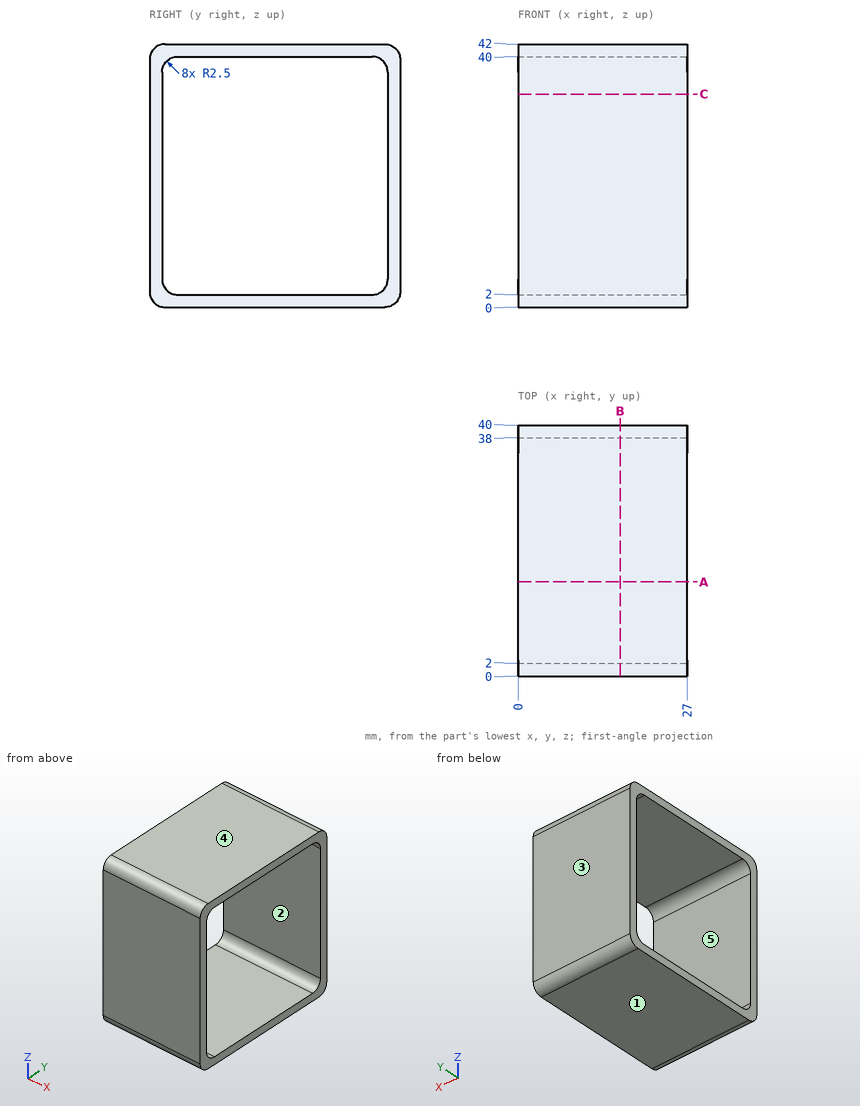
The figure shows three views and two pictorial views of one solid part (mm, origin at its lowest corner). Answer the questions. A direction names the side the tool comes from. Give positions to 0.01 mm unless a question says otherwise; leave off trailing zeros. Loops run counter-clockwise (first coordinate to the right, second up) from the corner with the lowest first, then second, coordinate; pieces in that order, holes last. Notation, with made-up numbers: (27, 35.5) -> (45, 35.5) arc R22 cw to (45, 44.5) -> close; hole circle Ø1 at (1.25, 76.5). An arc over 180 degrees is marked (long way). Put each result on its own line as item: value. Start each with the question number.
Item 1: The part is cut by section C-C (z = 34). Give the vertices of the cut face in (x, y).
Item 2: This flat-tipped pin is pushed along its axis until it touches: P1, Ø8, axis at y = 7, z = 19, coming from the -X side. Where does it stop, or does it pass through?
Item 3: Which of the six approach directions +Z, -Z, +X, -X, +Y, -Y give full straight-line access (tool end or side, diameter ignored) to the marked faces 4 and 5?
Item 4: The mould has two halves that part along Y. Classify the marked faces 1, 2 and 3: released by +Y, released by -Y, zero draft, split by the parting line, or undercut.
Item 5: Find the intervals of material crossed by L1, parallel to Z at x = 3, y = 8.5; L2, parallel to Y at x = 6.75, z = 36; L3, parallel to Y at x = 24.25, z = 39, in increasing order. Write a range as [from, to].
Item 6: The part is cut by section A-A (y = 15). Give the vertices of the cut face in (x, z).
Item 7: The part is cut by section B-B (x = 16.25). Give the vertices of the cut face in (y, z).
Answers below:
1. outline: (0, 0) -> (27, 0) -> (27, 2) -> (0, 2) -> close; (0, 38) -> (27, 38) -> (27, 40) -> (0, 40) -> close
2. P1: through
3. face 4: +Z, +X, -X, +Y, -Y
3. face 5: +X, -X
4. face 1: zero draft
4. face 2: undercut
4. face 3: released by +Y
5. L1: [0, 2], [40, 42]
5. L2: [0, 2], [38, 40]
5. L3: [0, 2.5], [37.5, 40]
6. outline: (0, 0) -> (27, 0) -> (27, 2) -> (0, 2) -> close; (0, 40) -> (27, 40) -> (27, 42) -> (0, 42) -> close
7. outline: (0, 2.5) arc R2.5 ccw to (2.5, 0) -> (37.5, 0) arc R2.5 ccw to (40, 2.5) -> (40, 39.5) arc R2.5 ccw to (37.5, 42) -> (2.5, 42) arc R2.5 ccw to (0, 39.5) -> close; hole (2, 4.5) arc R2.5 ccw to (4.5, 2) -> (35.5, 2) arc R2.5 ccw to (38, 4.5) -> (38, 37.5) arc R2.5 ccw to (35.5, 40) -> (4.5, 40) arc R2.5 ccw to (2, 37.5) -> close
